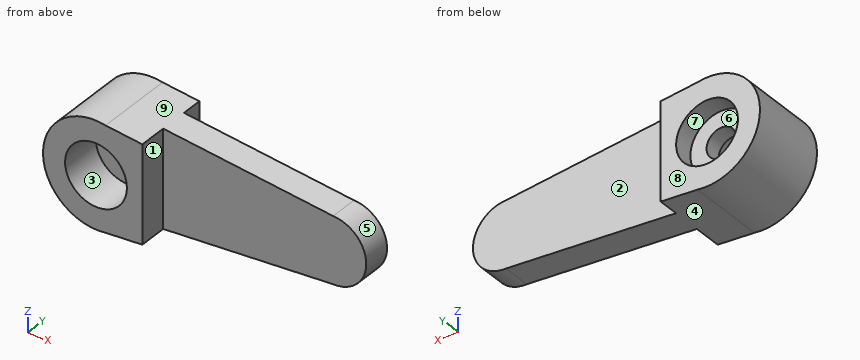
from build123d import *

# Parameters (mm, degrees)
SALIENTE_EXTRUIR2_DEPTH = 2.6
CROQUIS3_R              = 2.1
CORTAR_EXTRUIR1_DEPTH   = 1.3
CROQUIS5_R              = 1
CORTAR_EXTRUIR2_DEPTH   = 5
CORTAR_EXTRUIR3_START   = -2.8
CROQUIS6_R              = 2.1
CORTAR_EXTRUIR3_DEPTH   = 2.8
CROQUIS7_W              = 13.8
CROQUIS7_H              = 1.9
CORTAR_EXTRUIR4_DEPTH   = 5
CROQUIS10_W             = 13.8
CROQUIS10_H             = 2.15
CORTAR_EXTRUIR6_DEPTH   = 5


with BuildPart() as part:
    # Croquis1 → Saliente-Extruir2 (new, symmetric)
    with BuildSketch(Plane(origin=(0, 0, 0), x_dir=(1, 0, 0), z_dir=(0, 1, 0))):
        with BuildLine():
            Line((14.7, 2.25), (0.655694373, 3.53978317))
            ThreePointArc((0.655694373, 3.53978317), (-3.6, 0), (0.655694373, -3.53978317))
            Line((0.655694373, -3.53978317), (14.7, -2.25))
            ThreePointArc((14.7, -2.25), (16.95, 0), (14.7, 2.25))
        make_face()
    extrude(amount=SALIENTE_EXTRUIR2_DEPTH, both=True)

    # Croquis3 → Cortar-Extruir1 (cut)
    with BuildSketch(Plane(origin=(0, 2.6, 0), x_dir=(1, 0, 0), z_dir=(0, 1, 0))):
        with Locations(Location((0, 0, 0), (0, 0, 270))):
            Circle(CROQUIS3_R)
    extrude(amount=-CORTAR_EXTRUIR1_DEPTH, mode=Mode.SUBTRACT)

    # Croquis5 → Cortar-Extruir2 (cut)
    with BuildSketch(Plane(origin=(0, 1.3, 0), x_dir=(1, 0, 0), z_dir=(0, 1, 0))):
        with Locations(Location((0, 0, 0), (0, 0, 270))):
            Circle(CROQUIS5_R)
    extrude(amount=-CORTAR_EXTRUIR2_DEPTH, mode=Mode.SUBTRACT)

    # Croquis6 → Cortar-Extruir3 (cut)
    with BuildSketch(Plane.XZ.offset(2.6).offset(CORTAR_EXTRUIR3_START)):
        with Locations(Location((0, 0, 0), (0, 0, 90))):
            Circle(CROQUIS6_R)
    extrude(amount=CORTAR_EXTRUIR3_DEPTH, mode=Mode.SUBTRACT)

    # Croquis7 → Cortar-Extruir4 (cut, symmetric)
    with BuildSketch(Plane.XY):
        with Locations((10.05, -1.65)):
            Rectangle(CROQUIS7_W, CROQUIS7_H)
    extrude(amount=CORTAR_EXTRUIR4_DEPTH, both=True, mode=Mode.SUBTRACT)

    # Croquis10 → Cortar-Extruir6 (cut, symmetric)
    with BuildSketch(Plane.XY):
        with Locations((10.05, 2.274888949)):
            Rectangle(CROQUIS10_W, CROQUIS10_H)
    extrude(amount=CORTAR_EXTRUIR6_DEPTH, both=True, mode=Mode.SUBTRACT)


solid = part.part
Geometry: final body of the model. Coordinates: model frame, mm. Face numbers are marked on the shaded views. A direction names the side the tool comes from. Give positions to 0.01 mm unless a question says otherwise; leave off trailing zeros. Write each loop counter-clockwise with the first axis right and the second up, starting at its lowest first coordinate (ties: lowest second). Pieces come first, ordered by that corner, then holes. Notation, with made-up numbers: (0, 55) - (37, 55) arc R23 ccw to (37, 74) - close; hole circle Ø3 at (63.25, 29.25). An arc over 180 degrees is marked (long way). Return JSON: item names as keys, results as strings. Group by question number.
1) Section B-B on z = 0. Return the cut outline in (x, y).
2) Line query: line 1 (X direction, y = 0.65, z = 0); line 2 (Y direction, x = 11, z = -0.75); line 3 (Z direction, x = -0.5, y = -0.25). Output: solid intervals per line, ascending.
3) Section A-A on x = 0. Return the cut outline in (y, z), plus the area to 3 significant figures.
4) Section D-D on z = 2.5. Return the cut outline in (x, y), plus the area to 3 significant figures.
5) Set-up query: the marked faces 1, 2, 3, 4 and 5. Return all of +Z, -Z, +X, -X, +Y, -Y with unobstructed straight access to the full face (end or side cutting, diameter ignored); none if empty.
6) Section C-C on y = -2.1. Return the cut outline in (x, z), plus the area to 3 significant figures.
7) Mould query, pull axis Z, two halves, no side actions, for the marked faces 6, 7, 8 and 9. Classes: released by +Z, released by -Z, zero draft, split by the parting line, or undercut.
8) First-contact query: P1, Ø1.5, axis at x = 4.5, y = 1.5, coming from the -Z side; P2, Ø3, axis at x = 0, z = 0, coming from the -Y side; P3, Ø1, axis at x = 12.5, z = -1, coming from the -Y side. Flat tips, straight axial feed; report the tip coordinate or a pass-through.
Filled in:
{
 "1": {"outline": "(-3.6, -2.6) - (-2.1, -2.6) - (-2.1, 0.2) - (-1, 0.2) - (-1, 1.3) - (-2.1, 1.3) - (-2.1, 2.6) - (-3.6, 2.6) - close; (1, 0.2) - (2.1, 0.2) - (2.1, -2.6) - (3.15, -2.6) - (3.15, -0.7) - (16.95, -0.7) - (16.95, 1.2) - (3.15, 1.2) - (3.15, 2.6) - (2.1, 2.6) - (2.1, 1.3) - (1, 1.3) - close"},
 "2": {"line 1": "x = -3.6 to -1, 1 to 16.95", "line 2": "y = -0.7 to 1.2", "line 3": "z = -3.57 to -2.04, 2.04 to 3.57"},
 "3": {"outline": "(-2.6, -3.6) - (2.6, -3.6) - (2.6, -2.1) - (1.3, -2.1) - (1.3, -1) - (0.2, -1) - (0.2, -2.1) - (-2.6, -2.1) - close; (-2.6, 2.1) - (0.2, 2.1) - (0.2, 1) - (1.3, 1) - (1.3, 2.1) - (2.6, 2.1) - (2.6, 3.6) - (-2.6, 3.6) - close", "area": "18.0 mm^2"},
 "4": {"outline": "(-2.59, -2.6) - (3.15, -2.6) - (3.15, -0.7) - (11.98, -0.7) - (11.98, 1.2) - (3.15, 1.2) - (3.15, 2.6) - (-2.59, 2.6) - close", "area": "46.6 mm^2"},
 "5": {"face 1": "+Z, -Z, +X, -Y", "face 2": "+Z, -Z, +X, +Y", "face 3": "-Y", "face 4": "-Z, +X, +Y, -Y", "face 5": "+X, +Y, -Y"},
 "6": {"outline": "(0.66, -3.54) - (3.15, -3.31) - (3.15, 3.31) - (0.66, 3.54) arc R3.6 ccw (long way) to start; hole circle Ø4.2 at (0, 0)", "area": "28.3 mm^2"},
 "7": {"face 6": "undercut", "face 7": "undercut", "face 8": "zero draft", "face 9": "released by +Z"},
 "8": {"P1": "stops at z = -3.25", "P2": "stops at y = 0.2", "P3": "stops at y = -0.7"}
}
